CAD build for the part. Positions are in the model's coordinates, mm. Face numbers are marked on the shaded views. A direction names the side the tool comes from. Round coordinates to 2 decimals unless told otherwise and drop trailing zeros. Loops run counter-clockwise (first coordinate to the right, second up) from the corner with the lowest first, then second, coordinate; pieces in that order, holes last. Notation, with made-up numbers: (20.5, -22.5) - (32.5, -22.5) arc R21 cw to (32.5, -13.5) - close; hole circle Ø1 at (1, 26.5). An arc over 180 degrees is marked (long way). One line per question, with ' | ' between items.
```python
from build123d import *

# Parameters (mm, degrees)
EXTRUDE_1_DEPTH     = 16
CUT_EXTRUDE_1_DEPTH = 3


with BuildPart() as part:
    # 草图1 → 凸台-拉伸1 (new, symmetric)
    with BuildSketch(Plane.XY):
        with BuildLine():
            Line((-18, 0), (18, 0))
            Line((18, 0), (18, -7))
            Line((18, -7), (17, -7))
            Line((17, -7), (17, -24))
            Line((17, -24), (7.551896681, -24))
            Line((7.551896681, -24), (3, -18.575260778))
            ThreePointArc((3, -18.575260778), (0, -8.115719133), (-3, -18.575260778))
            Line((-3, -18.575260778), (-7.551896681, -24))
            Line((-7.551896681, -24), (-17, -24))
            Line((-17, -24), (-17, -7))
            Line((-17, -7), (-18, -7))
            Line((-18, -7), (-18, 0))
        make_face()
    extrude(amount=EXTRUDE_1_DEPTH, both=True)

    # 草图2 → 切除-拉伸1 (cut)
    with BuildSketch(Plane.XY.offset(16)):
        with BuildLine():
            Line((-7.551896681, -24), (-5.866143417, -21.990997492))
            ThreePointArc((-5.866143417, -21.990997492), (0, -5.306607169), (5.866143417, -21.990997492))
            Line((5.866143417, -21.990997492), (7.551896681, -24))
            ThreePointArc((7.551896681, -24), (0, -2.604245979), (-7.551896681, -24))
        make_face()
    extrude(amount=-CUT_EXTRUDE_1_DEPTH, mode=Mode.SUBTRACT)

    # 草图4 → M4 螺纹孔的螺纹孔钻头1 (revolve, cut)
    with BuildSketch(Plane(origin=(-12.5, 0, 10), x_dir=(0, 0, 1), z_dir=(1, 0, 0))):
        Polygon((0, 0), (0, 10.991420021), (1.65, 10), (1.65, 0), align=None)
    hole_wizard_m4_1 = revolve(axis=Axis((-12.5, 6.35, 10), (0, -1, 0)), mode=Mode.SUBTRACT)

    # 镜向1: M4 螺纹孔的螺纹孔钻头1 across plane
    add(hole_wizard_m4_1.mirror(Plane.XY), mode=Mode.SUBTRACT)

    # 镜向2: M4 螺纹孔的螺纹孔钻头1 across plane
    add(hole_wizard_m4_1.mirror(Plane(origin=(0, 0, 0), x_dir=(0, 0, 1), z_dir=(1, 0, 0))), mode=Mode.SUBTRACT)

    # 镜向2 copy 1 sketch → 镜向2 copy 1 (revolve, cut)
    with BuildSketch(Plane(origin=(12.5, 0, -10), x_dir=(0, 0, -1), z_dir=(-1, 0, 0))):
        Polygon((0, 0), (0, 10.991420021), (1.65, 10), (1.65, 0), align=None)
    revolve(axis=Axis((12.5, 6.35, -10), (0, -1, 0)), mode=Mode.SUBTRACT)


solid = part.part
```
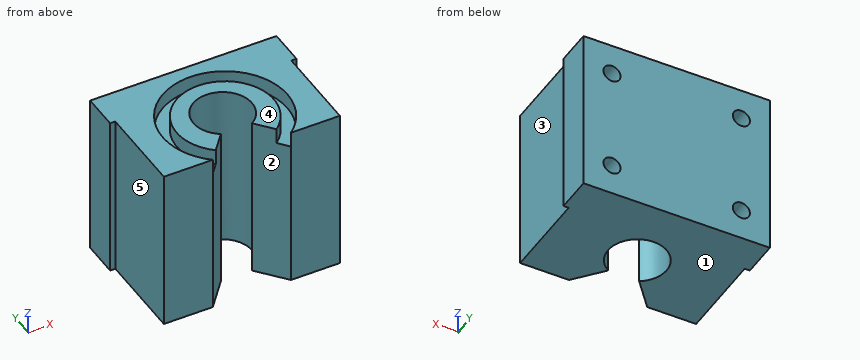
(1) Cut at C-C, the plane z = -13. Write the cut outline in (x, y).
Results found:
outline: (-18, -7) - (-17, -7) - (-17, -24) - (-7.55, -24) - (-3, -18.58) arc R5.66 cw (long way) to (3, -18.58) - (7.55, -24) - (17, -24) - (17, -7) - (18, -7) - (18, 0) - (-18, 0) - close
(2) Tool access for the marked faces 4 and 5: list every direction of +Z, -Z, +X, -X, +Y, -Y with a clear straight run to the whole face (end or side of a thin tool).
Results found:
face 4: +Z, +X, -X, +Y, -Y | face 5: +Z, -Z, -X, -Y
(3) Cut at B-B, the plane y = -11.5. Write the cut outline in (x, z).
Results found:
outline: (-17, -16) - (-5.18, -16) - (-5.18, 16) - (-8.82, 16) - (-8.82, 13) - (-11.62, 13) - (-11.62, 16) - (-17, 16) - close; (5.18, -16) - (17, -16) - (17, 16) - (11.62, 16) - (11.62, 13) - (8.82, 13) - (8.82, 16) - (5.18, 16) - close
(4) Probe L1, parallel to X at y = -2.5, z = 10; L2, parallel to X at y = -7.5, z = -10; L3, parallel to Z at x = -12.5, y = -3.5. List the from-to ranges inside material, lowest first.
Results found:
L1: x = -18 to -14.15, -10.85 to 10.85, 14.15 to 18 | L2: x = -17 to -14.15, -10.85 to 10.85, 14.15 to 17 | L3: z = -16 to -11.65, -8.35 to 8.35, 11.65 to 16
(5) Two-plate mould, pull along X, no slides. Class the marked faces 1, 2 and 3: released by +X, released by -X, zero draft, split by the parting line, or undercut.
Results found:
face 1: zero draft | face 2: undercut | face 3: released by +X
(6) Cut at D-D, the plane y = -16. Write the cut outline in (x, z).
Results found:
outline: (-17, -16) - (-5.2, -16) - (-5.2, 16) - (-9.28, 16) - (-9.28, 13) - (-11.95, 13) - (-11.95, 16) - (-17, 16) - close; (5.2, -16) - (17, -16) - (17, 16) - (11.95, 16) - (11.95, 13) - (9.28, 13) - (9.28, 16) - (5.2, 16) - close
(7) Cut at A-A, the plane x = 0. Write the cut outline in (y, z), then the cut area to 3 significant figures.
Results found:
outline: (-8.12, -16) - (0, -16) - (0, 16) - (-2.6, 16) - (-2.6, 13) - (-5.31, 13) - (-5.31, 16) - (-8.12, 16) - close | area: 252 mm²
(8) Drop flat-ended pins along their axis: P1, Ø2, axis at y = -13.5, z = -10.5, coming from the -X side; P2, Ø5, axis at x = 5, z = 9.5, coming from the -Y side; P3, Ø2.5, axis at x = -12.5, z = -10, coming from the +Y side. Give the stop position or say it passes through.
Results found:
P1: stops at x = -17 | P2: stops at y = -23.94 | P3: stops at y = -10.24
